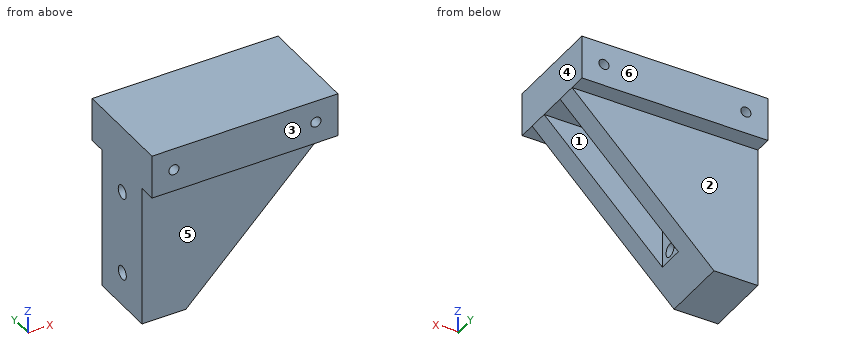
from build123d import *

# Parameters (mm, degrees)
PAD_DEPTH     = 20
SKETCH001_W   = 42
SKETCH001_H   = 8
POCKET_DEPTH  = 35
SKETCH002_R   = 2
HOLE_DEPTH    = 25
SKETCH003_R   = 1.5
HOLE001_DEPTH = 25
SKETCH004_W   = 55
SKETCH004_H   = 13
SKETCH004_R   = 1.5
PAD001_DEPTH  = 5
SKETCH005_W   = 55
SKETCH005_H   = 13
SKETCH005_R   = 1.5
PAD002_DEPTH  = 5


with BuildPart() as part:
    # Sketch → Pad (new body)
    with BuildSketch(Plane.XZ):
        Polygon((0, 0), (0, 55), (55, 55), (55, 42), (13, 0), align=None)
    extrude(amount=PAD_DEPTH)

    # Sketch001 (on Face3 of Pad) → Pocket (cut)
    with BuildSketch(Plane(origin=(55, 0, 0), x_dir=(0, 0, 1), z_dir=(1, 0, 0))):
        with Locations((21, 10)):
            Rectangle(SKETCH001_W, SKETCH001_H)
    extrude(amount=-POCKET_DEPTH, mode=Mode.SUBTRACT)

    # Sketch002 (on Face9 of Pocket) → Hole (cut)
    with BuildSketch(Plane(origin=(20, 0, 0), x_dir=(0, 0, 1), z_dir=(1, 0, 0))):
        with Locations((10, 10.133)):
            Circle(SKETCH002_R)
        with Locations((35, 10.080937)):
            Circle(SKETCH002_R)
    extrude(amount=-HOLE_DEPTH, mode=Mode.SUBTRACT)

    # Sketch003 (on Face4 of Hole) → Hole001 (cut)
    with BuildSketch(Plane.XZ.offset(20)):
        with Locations((6.5, 48.5)):
            Circle(SKETCH003_R)
        with Locations((48.5, 48.5)):
            Circle(SKETCH003_R)
    extrude(amount=-HOLE001_DEPTH, mode=Mode.SUBTRACT)

    # Sketch004 (on Face3 of Hole001) → Pad001 (join)
    with BuildSketch(Plane(origin=(0, 0, 0), x_dir=(1, 0, 0), z_dir=(0, 1, 0))):
        with Locations((27.5, -48.5)):
            Rectangle(SKETCH004_W, SKETCH004_H)
        with Locations((6.5, -48.5)):
            Circle(SKETCH004_R, mode=Mode.SUBTRACT)
        with Locations((48.5, -48.5)):
            Circle(SKETCH004_R, mode=Mode.SUBTRACT)
    extrude(amount=PAD001_DEPTH)

    # Sketch005 (on Face3 of Pad001) → Pad002 (join)
    with BuildSketch(Plane.XZ.offset(20)):
        with Locations((27.5, 48.5)):
            Rectangle(SKETCH005_W, SKETCH005_H)
        with Locations((6.5, 48.5)):
            Circle(SKETCH005_R, mode=Mode.SUBTRACT)
        with Locations((48.5, 48.5)):
            Circle(SKETCH005_R, mode=Mode.SUBTRACT)
    extrude(amount=PAD002_DEPTH)


solid = part.part
Part model, mm, in its own coordinate system. Face numbers are marked on the shaded views. A direction names the side the tool comes from. Coordinates: 2 decimals unless noted, no trailing zeros. Order: outer loops, then holes, each group sorted by start corner. A loop starts at its lowest first (then second) coordinate and runs counter-clockwise, first axis right, second up. Notation, with made-up numbers: M 88,-31 L 106,-31 A14 cw 106,-16 Z; hole C -23.5,50 d4. An arc over 180 degrees is marked long. Use a Markdown table: item, result.
(1) Tool access for the marked faces 5 and 6: list every direction of +Z, -Z, +X, -X, +Y, -Y with a clear straight run to the whole face (end or side of a thin tool).
A:
| item | result |
|---|---|
| face 5 | -Z, +X, -X, -Y |
| face 6 | +Z, -Z, +X, -X, +Y |
(2) Cut at A-A on z = 48.5. Write the cut outline in (x, y).
A:
| item | result |
|---|---|
| outline | M 0,-25 L 5,-25 L 5,5 L 0,5 Z; M 8,-25 L 47,-25 L 47,5 L 8,5 Z; M 50,-25 L 55,-25 L 55,5 L 50,5 Z |
(3) Cut at D-D on y = -3. Write the cut outline in (x, z).
A:
| item | result |
|---|---|
| outline | M 0,0 L 13,0 L 55,42 L 55,55 L 0,55 Z; hole C 6.5,48.5 d3; hole C 48.5,48.5 d3 |
(4) Pull direction Y, two halves, no side cores. Call the marked faces 1, 2, 3 and 4: released by +Y, released by -Y, zero draft, split by the parting line, or undercut.
A:
| item | result |
|---|---|
| face 1 | undercut |
| face 2 | released by +Y |
| face 3 | released by -Y |
| face 4 | zero draft |
(5) Cut at C-C on z = 35. Write the cut outline in (x, y).
A:
| item | result |
|---|---|
| outline | M 0,-20 L 48,-20 L 48,-14 L 20,-14 L 20,-12.08 L 0,-12.08 Z; M 0,-8.08 L 20,-8.08 L 20,-6 L 48,-6 L 48,0 L 0,0 Z |
(6) Flat gauge pins, fed straight in: pin 1 (12.5 mm diameter, centred on x = 20, z = 31.5, fed in from +Y); pin 2 (5.5 mm diameter, centred on x = 20.5, y = -22, fed in from -Z); pin 3 (5 mm diameter, centred on y = -10.133, z = 10, fed in from +X). Where does each tip first touch, or does it go through?
A:
| item | result |
|---|---|
| pin 1 | stops at y = 0 |
| pin 2 | stops at z = 5.61 |
| pin 3 | stops at x = 20 |
(7) Cut at B-B on x = 7. Write the cut outline in (y, z).
A:
| item | result |
|---|---|
| outline | M -25,42 L -20,42 L -20,0 L 0,0 L 0,42 L 5,42 L 5,47.09 L -25,47.09 Z; M -25,49.91 L 5,49.91 L 5,55 L -25,55 Z; hole C -10.13,10 d4; hole C -10.08,35 d4 |
(8) Probe L1, parallel to X at y = -8.5, z = 48.5; L2, parallel to Y at x = 6, z = 10; L3, parallel to Y at x = 31.5, z = 39. List the from-to ranges inside material, lowest first.
A:
| item | result |
|---|---|
| L1 | x = 0 to 5, 8 to 47, 50 to 55 |
| L2 | y = -20 to -12.13, -8.13 to 0 |
| L3 | y = -20 to -14, -6 to 0 |
